```python
from build123d import *

# Parameters (mm, degrees)
BOSS_EXTRUDE1_DEPTH = 9.5
SHELL1_T            = -1.5
FILLET2_R           = 0.5
SKETCH2_R           = 4.75
BOSS_EXTRUDE2_DEPTH = 8
SKETCH4_R           = 3.1
BOSS_EXTRUDE3_DEPTH = 17.8
SKETCH5_R           = 5
SKETCH5_R_2         = 2.15
CUT_EXTRUDE1_DEPTH  = 1.7
CHAMFER1_SIZE       = 1


with BuildPart() as part:
    # Sketch1 → Boss-Extrude1 (new body)
    with BuildSketch(Plane.XY):
        with BuildLine():
            ThreePointArc((2.992904177, 11.872881569), (0, 14.666666667), (-2.992904177, 11.872881569))
            ThreePointArc((-2.992904177, 11.872881569), (-5.625090617, 3.247647582), (-11.778669143, -3.344509736))
            ThreePointArc((-11.778669143, -3.344509736), (-12.701705922, -7.333333333), (-8.785764966, -8.528371833))
            ThreePointArc((-8.785764966, -8.528371833), (0, -6.495295163), (8.785764966, -8.528371833))
            ThreePointArc((8.785764966, -8.528371833), (12.701705922, -7.333333333), (11.778669143, -3.344509736))
            ThreePointArc((11.778669143, -3.344509736), (5.625090617, 3.247647582), (2.992904177, 11.872881569))
        make_face()
    extrude(amount=BOSS_EXTRUDE1_DEPTH)

    # Shell1
    shell1_openings = [part.faces().sort_by_distance(p)[0] for p in [
        (0, 0, 9.5),
    ]]
    offset(amount=SHELL1_T, openings=shell1_openings, kind=Kind.INTERSECTION)

    # Fillet2
    fillet2_edges = [part.edges().sort_by_distance(p)[0] for p in [
        (-12.701705922, -7.333333333, 0),
        (-5.625090617, 3.247647582, 0),
        (0, 14.666666667, 0),
        (5.625090617, 3.247647582, 0),
        (12.701705922, -7.333333333, 0),
        (0, -6.495295163, 0),
    ]]
    fillet(fillet2_edges, radius=FILLET2_R)

    # Sketch2 → Boss-Extrude2 (add)
    with BuildSketch(Plane.XY.offset(1.5)):
        Circle(SKETCH2_R)
    extrude(amount=BOSS_EXTRUDE2_DEPTH)

    # Sketch4 → Boss-Extrude3 (add)
    with BuildSketch(Plane.XY.offset(9.5)):
        Circle(SKETCH4_R)
    extrude(amount=BOSS_EXTRUDE3_DEPTH)

    # Sketch5 → Cut-Extrude1 (cut)
    with BuildSketch(Plane.XY.offset(20.8)):
        Circle(SKETCH5_R)
        Circle(SKETCH5_R_2, mode=Mode.SUBTRACT)
    extrude(amount=-CUT_EXTRUDE1_DEPTH, mode=Mode.SUBTRACT)

    # Chamfer1
    chamfer1_edges = [part.edges().sort_by_distance(p)[0] for p in [
        (-3.1, 0, 27.3),
    ]]
    chamfer(chamfer1_edges, length=CHAMFER1_SIZE)


solid = part.part
```
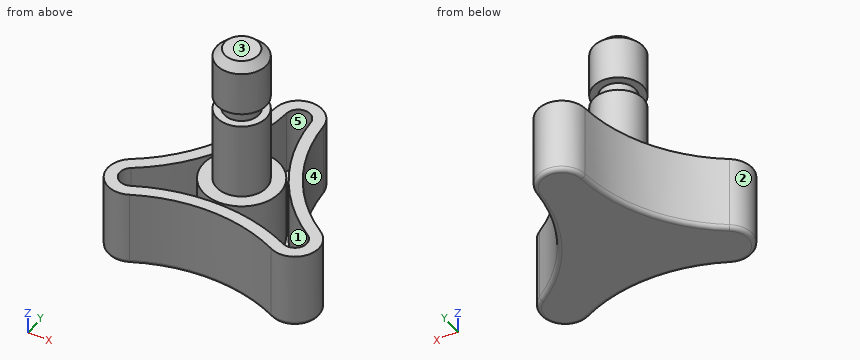
Work out the finished part from the listing and answer in its coordinate system (mm). Face numbers are marked on the shaded views. A direction names the side the tool comes from. Give positions to 0.01 mm unless a question says otherwise; leave off trailing zeros. Loops run counter-clockwise (first coordinate to the right, second up) from the corner with the lowest first, then second, coordinate; pieces in that order, holes last. Notation, with made-up numbers: (-16, 40.25) -> (37, 40.25) arc R7 ccw to (37, 52.25) -> close; hole circle Ø11 at (71, 17). An arc over 180 degrees is marked (long way). One line per question, with ' | ' between items. Start each with the question number.
1) Determine the mould class of the marked faces 1, 2 and 3 for opening direction Y: +Y half, -Y half, draft (parallel to the pull), parting line (faces both ways), or undercut.
2) Section A-A, the plane z = 4.5 is taken. Determine the outline of the cut face in (x, y), then the cut area to 3 significant figures.
3) Straight lines are drawn through the part: L1, parallel to X at y = 1.5, z = 9; L2, parallel to Z at x = -2.5, y = 4; L3, parallel to X at y = -0.75, z = 8. For each, find the intervals that lie inside material, in ascending order.
4) Each of these flat-tipped pins is pushed along its axis until it touches: pin 1 (8 mm diameter, centred on y = 6, z = 17, fed in from +X); pin 2 (4 mm diameter, centred on x = -2, y = -3, fed in from +Z); pin 3 (1.5 mm diameter, centred on x = -4.5, y = 12, fed in from -Z); pin 4 (12 mm diameter, centred on y = -6, z = 18.5, fed in from -X). Where does it stop, or does it pass through?
5) For the marked faces 4 and 5, determine the directions among +Z, -Z, +X, -X, +Y, -Y from which every point of the face is accessible in a straight line to the end or side of a thin tool.
6) Section B-B, the plane x = 0 is taken. Determine the outline of the cut face in (y, z), then the cut area to 3 significant figures.
7) Section C-C, the plane z = 13 is taken. Determine the outline of the cut face in (x, y).
Resolved:
1) face 1: undercut | face 2: parting line | face 3: draft
2) outline: (-11.78, -3.34) arc R3 ccw to (-8.79, -8.53) arc R20 cw to (8.79, -8.53) arc R3 ccw to (11.78, -3.34) arc R20 cw to (2.99, 11.87) arc R3 ccw to (-2.99, 11.87) arc R20 cw to start; circle Ø9.5 at (0, 0); hole (-10.94, -4.59) arc R1.5 ccw to (-9.44, -7.18) arc R21.5 cw to (9.44, -7.18) arc R1.5 ccw to (10.94, -4.59) arc R21.5 cw to (1.5, 11.77) arc R1.5 ccw to (-1.5, 11.77) arc R21.5 cw to start | area: 186 mm2
3) L1: -6.76 to -4.94, -4.51 to 4.51, 4.94 to 6.76 | L2: 0 to 9.5 | L3: -8.66 to -6.63, -4.69 to 4.69, 6.63 to 8.66
4) pin 1: x = 2.37 | pin 2: z = 27.3 | pin 3: through | pin 4: x = -3.1
5) face 4: +Z, -Z, +X, +Y | face 5: +Z
6) outline: (-6.5, 0.5) arc R0.5 ccw to (-6, 0) -> (14.17, 0) arc R0.5 ccw to (14.67, 0.5) -> (14.67, 9.5) -> (13.17, 9.5) -> (13.17, 1.5) -> (4.75, 1.5) -> (4.75, 9.5) -> (3.1, 9.5) -> (3.1, 19.1) -> (2.15, 19.1) -> (2.15, 20.8) -> (3.1, 20.8) -> (3.1, 26.3) -> (2.1, 27.3) -> (-2.1, 27.3) -> (-3.1, 26.3) -> (-3.1, 20.8) -> (-2.15, 20.8) -> (-2.15, 19.1) -> (-3.1, 19.1) -> (-3.1, 9.5) -> (-4.75, 9.5) -> (-4.75, 1.5) -> (-5, 1.5) -> (-5, 9.5) -> (-6.5, 9.5) -> close | area: 238 mm2
7) outline: circle Ø6.2 at (0, 0)
